Verification items for the finished model (mm, model axes). Coordinates: 2 decimals unless noted, no trailing zeros. Order: outer loops, then holes, each group sorted by start corner. A loop starts at its lowest first (then second) coordinate and runs counter-clockwise, first axis right, second up. Notation, with made-up numbers: (-33.5, 39) -> (15.5, 39) arc R15 ccw to (15.5, 55) -> close; hole circle Ø8 at (89, -7). An arc over 180 degrees is marked (long way). Write item = value, one per line. Start each with the question number.
1. Cross-section at B-B on x = -12. Record the cut outline in (y, z).
2. Cross-section at C-C on y = -8.5. Record the cut outline in (x, z), plus the area to 3 significant figures.
3. Thickness scan on line 1 along X through (y, z) = (-4, 0.9); line 2 along X through (y, z) = (-7.5, 0.55); line 3 along Y through (x, z) = (6.5, 1.2). Record the ranges inside material, lowest first. Write a range as from..to.
4. Cross-section at A-A on z = 0.3. Record the cut outline in (x, y), plus the area to 3 significant figures.
from build123d import *

# Parameters (mm, degrees)
SKETCH_1_W      = 26.56
SKETCH_1_H      = 22
EXTRUDE_1_DEPTH = 2.2
FILLET_1_R      = 13.5


with BuildPart() as part:
    # Эскиз1 → Бобышка-Вытянуть1 (new body)
    with BuildSketch(Plane.XY):
        with Locations((-4.253421702, 0.2)):
            Rectangle(SKETCH_1_W, SKETCH_1_H)
    extrude(amount=EXTRUDE_1_DEPTH)

    # Скругление1
    # the kernel refuses this fillet: 13.5 mm, written as the material it takes off along each edge
    with BuildSketch(Plane(origin=(9.026578298, -10.8, -33.75), x_dir=(0, 1, 0), z_dir=(0, 0, 1)), Plane(origin=(-17.533421702, -10.8, -33.75), x_dir=(1, 0, 0), z_dir=(0, 0, 1))) as fillet_1_piece_1:
        with BuildLine():
            CenterArc((FILLET_1_R, FILLET_1_R), FILLET_1_R, 180, 90)
            Line((0, FILLET_1_R), (0, 0))
            Line((0, 0), (FILLET_1_R, 0))
        make_face()
    extrude(amount=69.7, mode=Mode.SUBTRACT)


solid = part.part
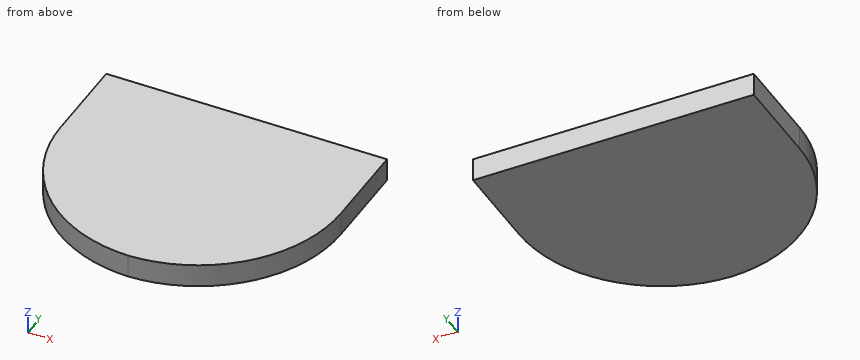
Worked out:
q1.outline = (-8.2, 0) -> (11.2, 0) -> (11.2, 2.2) -> (-8.2, 2.2) -> close
q2.outline = (-11.57, 0) -> (3.06, 0) -> (3.06, 2.2) -> (-11.57, 2.2) -> close
q2.area = 32.2 mm²
q3.line_1 = -15.75..7.25
q3.line_2 = -12.88..4.37
q3.line_3 = -5.16..11.2
q4.outline = (-17.53, 2.7) arc R13.5 ccw to (-4.25, -10.8) arc R13.5 ccw to (9.03, 2.7) -> (9.03, 11.2) -> (-17.53, 11.2) -> close
q4.area = 506 mm²
